Part model, mm, in its own coordinate system. A direction names the side the tool comes from. Give positions to 0.01 mm unless a question says otherwise; leave off trailing zeros. Loops run counter-clockwise (first coordinate to the right, second up) from the corner with the lowest first, then second, coordinate; pieces in that order, holes last. Notation, with made-up numbers: M 18,49 L 56,49 A24 ccw 56,71 Z; hole C -36,-15.5 d1. An arc over 180 degrees is marked long. Answer in a Markdown table with one row per item.
from build123d import *

# Parameters (mm, degrees)
SKETCH1_W           = 48
SKETCH1_H           = 20
SKETCH1_R           = 6.1
SKETCH1_R_2         = 4.1
BOSS_EXTRUDE1_DEPTH = 30
SKETCH2_W           = 48
SKETCH2_H           = 20
BOSS_EXTRUDE2_DEPTH = 20
SKETCH3_R           = 6.1
CUT_EXTRUDE1_DEPTH  = 40


with BuildPart() as part:
    # Sketch1 → Boss-Extrude1 (new body)
    with BuildSketch(Plane.XY):
        Rectangle(SKETCH1_W, SKETCH1_H)
        with Locations((-14, 0)):
            Circle(SKETCH1_R, mode=Mode.SUBTRACT)
        with Locations((16, 0)):
            Circle(SKETCH1_R_2, mode=Mode.SUBTRACT)
    extrude(amount=BOSS_EXTRUDE1_DEPTH)

    # Sketch2 → Boss-Extrude2 (add)
    with BuildSketch(Plane(origin=(0, 0, 0), x_dir=(-1, 0, 0), z_dir=(0, 0, -1))):
        Rectangle(SKETCH2_W, SKETCH2_H)
    extrude(amount=BOSS_EXTRUDE2_DEPTH)

    # Sketch3 → Cut-Extrude1 (cut)
    with BuildSketch(Plane(origin=(24, 0, 0), x_dir=(0, 0, -1), z_dir=(1, 0, 0))):
        with Locations((10, 0)):
            Circle(SKETCH3_R)
    extrude(amount=-CUT_EXTRUDE1_DEPTH, mode=Mode.SUBTRACT)


solid = part.part
(1) Saw through at C-C (y = 0). Write the cut outline in (x, z).
Recorded:
| item | result |
|---|---|
| outline | M -24,-20 L 24,-20 L 24,-16.1 L -16,-16.1 L -16,-3.9 L 24,-3.9 L 24,30 L 20.1,30 L 20.1,0 L 11.9,0 L 11.9,30 L -7.9,30 L -7.9,0 L -20.1,0 L -20.1,30 L -24,30 Z |
(2) Pull direction Y, two halves, no side cores. Call faces 1 (the face through (11.904, 0.18, 14.79)), 2 (the face through (0, 10, 5)), 3 (the face through (24, 0, 5)): +Y half, -Y half, draft (parallel to the pull), parting line (faces both ways), or undercut.
Recorded:
| item | result |
|---|---|
| face 1 | undercut |
| face 2 | +Y half |
| face 3 | draft |
(3) Saw through at A-A (x = 16). Write the cut outline in (y, z).
Recorded:
| item | result |
|---|---|
| outline | M -10,-20 L 10,-20 L 10,30 L 4.1,30 L 4.1,0 L -4.1,0 L -4.1,30 L -10,30 Z; hole C 0,-10 d12.2 |
(4) Which spindle directions (+Z, -Z, +X, -X, +Y, -Y) get a long thin tool onto all of the face, cutting with end or side? Do faces 4 (the face through (-24, 0, 5)), 5 (the face through (-20.094, 0.268, 14.79)), 6 (the face through (-16, 0, -10)). Say none if no direction does.
Recorded:
| item | result |
|---|---|
| face 4 | +Z, -Z, -X, +Y, -Y |
| face 5 | +Z |
| face 6 | +X |
(5) Pin check, flat tip, straight feed: pin 1 Ø3.5 at (y, z) = (0, -7.5) entering from +X. Stop position of the tip, or through.
Recorded:
| item | result |
|---|---|
| pin 1 | stops at x = -16 |
(6) Drill centre lines: line 1 along Y through (x, z) = (10.5, -10); line 2 along Y through (x, z) = (16, 12); line 3 along X through (y, z) = (1.75, -10.5). Where is each one in solid material? Low to high.
Recorded:
| item | result |
|---|---|
| line 1 | y = -10 to -6.1, 6.1 to 10 |
| line 2 | y = -10 to -4.1, 4.1 to 10 |
| line 3 | x = -24 to -16 |
(7) Saw through at B-B (z = -10). Write the cut outline in (x, y).
Recorded:
| item | result |
|---|---|
| outline | M -24,-10 L 24,-10 L 24,-6.1 L -16,-6.1 L -16,6.1 L 24,6.1 L 24,10 L -24,10 Z |
(8) Saw through at D-D (x = -14). Write the cut outline in (y, z), plus the area to 3 significant figures.
Recorded:
| item | result |
|---|---|
| outline | M -10,-20 L 10,-20 L 10,30 L 6.1,30 L 6.1,0 L -6.1,0 L -6.1,30 L -10,30 Z; hole C 0,-10 d12.2 |
| area | 517 mm^2 |
